Input: part model. Units: mm. Frame: model coordinates. A direction names the side the tool comes from. Give positions to 0.01 mm unless a question says otherwise; leave off trailing zeros. Loops run counter-clockwise (first coordinate to the right, second up) from the corner with the lowest first, then second, coordinate; pieces in that order, holes last.
from build123d import *

# Parameters (mm, degrees)
F0_R     = 44.3
F0_R_2   = 43
F1_DEPTH = 6
F0_R_3   = 50
F2_DEPTH = 1.3
F0_R_4   = 4.5
F4_DEPTH = 39.7


with BuildPart() as f1:
    # F0 (on Top) → F1 (new body)
    with BuildSketch(Plane.XY):
        Circle(F0_R)
        Circle(F0_R_2, mode=Mode.SUBTRACT)
    extrude(amount=F1_DEPTH)

    # F0 (on Top) → F2 (join)
    with BuildSketch(Plane.XY):
        Circle(F0_R_3)
        Circle(F0_R, mode=Mode.SUBTRACT)
    extrude(amount=F2_DEPTH)



with BuildPart() as f2:
    # F0 (on Top) → F2, piece 2 (new body)
    with BuildSketch(Plane.XY):
        Circle(F0_R_4)
    extrude(amount=F2_DEPTH)


with BuildPart() as f1_1:
    add(f1.part)

    add(f2.part)  # F4 merges F2
    # F3 (on Top) → F4 (join)
    with BuildSketch(Plane.XY):
        with BuildLine():
            Line((0.813912513, 56.8630076668), (0, 57.7447935939))
            ThreePointArc((0, 57.7447935939), (-12.6366686131, 29.501028063), (-0.9101021846, 0.8674232463))
            ThreePointArc((-0.9101021846, 0.8674232463), (-0.7483916982, 0.9566019765), (-0.5871154535, 1.046563636))
            Line((-0.5871154535, 1.046563636), (0, 0))
            ThreePointArc((0, 0), (0.267331286, 0.5689785091), (0.5437314891, 1.1336071376))
            ThreePointArc((0.5437314891, 1.1336071376), (-11.4412500514, 29.057066575), (0.813912513, 56.8630076668))
        make_face()
        with BuildLine():
            ThreePointArc((-0.5871154535, 1.046563636), (-0.7483916982, 0.9566019765), (-0.9101021846, 0.8674232463))
            ThreePointArc((-0.9101021846, 0.8674232463), (-0.4585208082, 0.4300711904), (0, 0))
            Line((0, 0), (-0.5871154535, 1.046563636))
        make_face()
        with BuildLine():
            ThreePointArc((0, 0), (-0.4585208082, 0.4300711904), (-0.9101021846, 0.8674232463))
            ThreePointArc((-0.9101021846, 0.8674232463), (-31.1704532134, -1.9021480376), (-53.8284211792, 18.3457125195))
            Line((-53.8284211792, 18.3457125195), (-54.9185622296, 17.8441225572))
            ThreePointArc((-54.9185622296, 17.8441225572), (-31.9620903304, -2.9018670057), (-1.1062055724, -0.5975100887))
            ThreePointArc((-1.1062055724, -0.5975100887), (-1.1410482964, -0.4161565338), (-1.1767698186, -0.2349740286))
            Line((-1.1767698186, -0.2349740286), (0, 0))
        make_face()
        with BuildLine():
            ThreePointArc((0.5437314891, 1.1336071376), (0.267331286, 0.5689785091), (0, 0))
            Line((0, 0), (0.813912513, 0.8817859271))
            ThreePointArc((0.813912513, 0.8817859271), (0.67851679, 1.0073690689), (0.5437314891, 1.1336071376))
        make_face()
        with BuildLine():
            Line((-0.1401682913, -1.1917855722), (0, 0))
            ThreePointArc((0, 0), (-0.5507127301, -0.3031798959), (-1.1062055724, -0.5975100887))
            ThreePointArc((-1.1062055724, -0.5975100887), (-7.8231494792, -30.2326587139), (-34.0817063625, -45.5247337819))
            Line((-34.0817063625, -45.5247337819), (-33.9415380712, -46.7165193541))
            ThreePointArc((-33.9415380712, -46.7165193541), (-7.1169895626, -31.2944805034), (0.2264295423, -1.2367047898))
            ThreePointArc((0.2264295423, -1.2367047898), (0.0431850682, -1.213800859), (-0.1401682913, -1.1917855722))
        make_face()
        with BuildLine():
            Line((1.0901410504, -0.5015899623), (0, 0))
            ThreePointArc((0, 0), (0.118161623, -0.6174466707), (0.2264295423, -1.2367047898))
            ThreePointArc((0.2264295423, -1.2367047898), (26.3354809362, -16.7826626179), (32.7647682526, -46.4815453255))
            Line((32.7647682526, -46.4815453255), (33.9415380712, -46.7165193541))
            ThreePointArc((33.9415380712, -46.7165193541), (27.5635488832, -16.4391856056), (1.2461467256, -0.1668155054))
            ThreePointArc((1.2461467256, -0.1668155054), (1.1677381364, -0.3340136527), (1.0901410504, -0.5015899623))
        make_face()
        with BuildLine():
            ThreePointArc((-1.1062055724, -0.5975100887), (-0.5507127301, -0.3031798959), (0, 0))
            Line((0, 0), (-1.1767698186, -0.2349740286))
            ThreePointArc((-1.1767698186, -0.2349740286), (-1.1410482964, -0.4161565338), (-1.1062055724, -0.5975100887))
        make_face()
        with BuildLine():
            Line((0.813912513, 0.8817859271), (0, 0))
            ThreePointArc((0, 0), (0.6237406292, -0.0784231329), (1.2461467256, -0.1668155054))
            ThreePointArc((1.2461467256, -0.1668155054), (24.0993718078, 19.8604027943), (54.3314467761, 16.7975589211))
            Line((54.3314467761, 16.7975589211), (54.9185622296, 17.8441225572))
            ThreePointArc((54.9185622296, 17.8441225572), (24.152199623, 21.1345050517), (0.5437314891, 1.1336071376))
            ThreePointArc((0.5437314891, 1.1336071376), (0.67851679, 1.0073690689), (0.813912513, 0.8817859271))
        make_face()
        with BuildLine():
            ThreePointArc((0.2264295423, -1.2367047898), (0.118161623, -0.6174466707), (0, 0))
            Line((0, 0), (-0.1401682913, -1.1917855722))
            ThreePointArc((-0.1401682913, -1.1917855722), (0.0431850682, -1.213800859), (0.2264295423, -1.2367047898))
        make_face()
        with BuildLine():
            ThreePointArc((1.2461467256, -0.1668155054), (0.6237406292, -0.0784231329), (0, 0))
            Line((0, 0), (1.0901410504, -0.5015899623))
            ThreePointArc((1.0901410504, -0.5015899623), (1.1677381364, -0.3340136527), (1.2461467256, -0.1668155054))
        make_face()
    extrude(amount=F4_DEPTH)

    # F5 (on Right) → F6 (revolve, cut)
    with BuildSketch(Plane.YZ):
        with BuildLine():
            Line((64.435094595, 43.7389037002), (33.4996059537, 43.7389037002))
            ThreePointArc((33.4996059537, 43.7389037002), (52.6054366049, 37.5412075606), (64.435094595, 21.3084199335))
            Line((64.435094595, 21.3084199335), (64.435094595, 43.7389037002))
        make_face()
        with BuildLine():
            ThreePointArc((61.4731870592, 13.4233012795), (57.7598621582, 3.0573466208), (48.3091473579, -2.5929443073))
            Line((48.3091473579, -2.5929443073), (61.4731870592, -2.5929443073))
            Line((61.4731870592, -2.5929443073), (61.4731870592, 13.4233012795))
        make_face()
    revolve(axis=Axis((0, 0, 0), (0, 0, -1)), mode=Mode.SUBTRACT)


solid = f1_1.part
(1) Cut plane D-D (z = 37). Return the cut outline in (x, y), and give its area (3 significant figures).
Values follow:
outline: (-51.87, 12.4) arc R39.29 ccw to (-1.11, -0.6) arc R38.09 cw to (-29.2, -44.63) arc R53.33 ccw to (-27.82, -45.5) arc R39.29 ccw to (0.23, -1.24) arc R38.09 cw to (33.42, -41.56) arc R53.33 ccw to (34.67, -40.52) arc R39.29 ccw to (1.25, -0.17) arc R38.09 cw to (49.85, 18.94) arc R53.33 ccw to (49.25, 20.46) arc R39.29 ccw to (0.54, 1.13) arc R38.09 cw to (-2.61, 53.27) arc R53.33 ccw to (-4.23, 53.16) arc R39.29 ccw to (-0.91, 0.87) arc R38.09 cw to (-51.46, 13.98) arc R53.33 ccw to start
area: 348 mm2
(2) Ray query, probe 1 along Y at (x, z) = (-38, 4.5); probe 2 along X at (y, z) = (-24, 5.5); probe 3 along X at (y, z) = (6.5, 33.5). Return the intervals inside material, ascending.
Values follow:
probe 1: y = -22.77 to -20.12, -0.25 to 1.13, 20.12 to 22.77
probe 2: x = -37.24 to -35.68, -4.11 to -2.78, 30.41 to 31.72, 35.68 to 37.24
probe 3: x = -47.02 to -45.3, -5.65 to -4.18, 3.78 to 5.27
(3) Mould query, pull axis Y, two halves, no side actions, for faces 1 (the cylindrical face through (44.02, -4.98, 3.62)), 2 (the flat face through (-37, -23, 6)), 3 (the flat face through (-33, 31, 1.3)). Classes: +Y half, -Y half, draft (parallel to the pull), parting line (faces both ways), or undercut.
Values follow:
face 1: undercut
face 2: undercut
face 3: draft
(4) Cut plane A-A (y = -24). Return the cut outline in (x, z).
Values follow:
outline: (-43.86, 0) - (-35.68, 0) - (-35.68, 6) - (-37.24, 6) - (-37.24, 1.3) - (-43.86, 1.3) - close; (-4.11, 0) - (-2.78, 0) - (-2.78, 39.7) - (-4.11, 39.7) - close; (30.41, 0) - (31.72, 0) - (31.72, 39.7) - (30.41, 39.7) - close; (35.68, 0) - (43.86, 0) - (43.86, 1.3) - (37.24, 1.3) - (37.24, 6) - (35.68, 6) - close
(5) Cut plane C-C (x = 22.5). Return the cut outline in (y, z).
Values follow:
outline: (-44.65, 0) - (-36.64, 0) - (-36.64, 6) - (-38.16, 6) - (-38.16, 1.3) - (-44.65, 1.3) - close; (-12.24, 0) - (-10.56, 0) - (-10.56, 39.7) - (-12.24, 39.7) - close; (19.31, 0) - (20.59, 0) - (20.59, 39.7) - (19.31, 39.7) - close; (36.64, 0) - (44.65, 0) - (44.65, 1.3) - (38.16, 1.3) - (38.16, 6) - (36.64, 6) - close
(6) Cut plane B-B (z = 19.5). Return the cut outline in (x, y), and give its area (3 significant figures).
Values follow:
outline: (-54.92, 17.84) arc R39.29 ccw to (-1.11, -0.6) arc R38.09 cw to (-34.08, -45.52) - (-33.94, -46.72) arc R39.29 ccw to (0.23, -1.24) arc R38.09 cw to (32.76, -46.48) - (33.94, -46.72) arc R39.29 ccw to (1.25, -0.17) arc R38.09 cw to (54.33, 16.8) - (54.92, 17.84) arc R39.29 ccw to (0.54, 1.13) arc R38.09 cw to (0.81, 56.86) - (0, 57.74) arc R39.29 ccw to (-0.91, 0.87) arc R38.09 cw to (-53.83, 18.35) - close
area: 382 mm2
(7) Reachability of faces 4 (the cylindrical face through (26.08, -16.43, 19.57)), 5 (the flat face through (18, 40, 6)), 6 (the cylindrical face through (-2.65, -3.637, 0.641)) from +Z, -Z, +X, -X, +Y, -Y: full face, straight path, thin tool, end or side. Return the list, or none.
Values follow:
face 4: +Z
face 5: +Z, +X
face 6: +Z, -Z
(8) Pin query (flat end, axial travel): pin 1 Ø8 at (x, y) = (2, 40.5) entering from +Z; pin 2 Ø4 at (x, y) = (-3, -2) entering from +Z; pin 3 Ø10 at (y, z) = (-24.5, 9) entering from -X; pin 4 Ø1 at (y, z) = (-34.5, 22) entering from +X. Return the tip coordinate at first contact, or that it passes through.
Values follow:
pin 1: stops at z = 6
pin 2: stops at z = 39.7
pin 3: stops at x = -39.27
pin 4: stops at x = 34.5
